Check sheet for the modelled part. Datum: model origin and axes. Units: mm. A direction names the side the tool comes from. Coordinates: 2 decimals unless noted, no trailing zeros. Loops run counter-clockwise (first coordinate to the right, second up) from the corner with the lowest first, then second, coordinate; pieces in that order, holes last. Notation, with made-up numbers: (-1, 32.25) - (8, 32.25) arc R29 cw to (8, 66.25) - close; hole circle Ø5 at (15, 75). An arc over 180 degrees is marked (long way). Write each question's results on one line, items separated by ' | '. Start each with the question number.
1. Gauge pin test, flat ends, axial feed: P1, Ø6, axis at x = 4.5, z = 14.5, coming from the +Y side; P2, Ø8, axis at x = 7.5, y = -7, coming from the +Z side; P3, Ø12, axis at x = 5, y = -9.5, coming from the -Z side. Record the tip position at first contact, or that the pin passes through.
2. Tool access check on faces 1 (the face through (11, 18, 40)), 2 (the face through (7.385, 0.751, -3.698)). Record the directions out of +Z, -Z, +X, -X, +Y, -Y that give a thin tool (end or side, any length) a straight path to the whole face; none if there is none.
3. Thickness scan on line 1 (Z direction, x = -13, y = 6.5); line 2 (Z direction, x = 7, y = 9); line 3 (X direction, y = 0.5, z = 20). Record the ranges inside material, lowest first. Write a range as [from, to].
4. Cross-section at B-B (z = 19). Record the cut outline in (x, y), and give its area (3 significant figures).
5. Cross-section at A-A (z = -3). Record the cut outline in (x, y), and give its area (3 significant figures).
```python
from build123d import *


with BuildPart() as f1:
    # F0 (on Front) → F1 (revolve)
    with BuildSketch(Plane.XZ):
        Polygon((10, 35), (5, 35), (5, -7.5), (7.5, -7.5), (7.5, 0), (10, 0), align=None)
        with BuildLine():
            Line((5, 37), (5, 35))
            Line((5, 35), (10, 35))
            Line((10, 35), (25, 35))
            Line((25, 35), (25, 40))
            Line((25, 40), (23.734994, 40))
            ThreePointArc((23.734994, 40), (14.486833, 37.754747), (5, 37))
        make_face()
    revolve(axis=Axis((5, 0, 14.75), (0, 0, 1)))


solid = f1.part
```
Established:
1) P1: y = 5 | P2: z = 38.1 | P3: z = 0
2) face 1: +Z, +X, -X, +Y, -Y | face 2: -Z
3) line 1: [35, 40] | line 2: [35, 37.71] | line 3: [0.03, 9.97]
4) outline: circle Ø10 at (5, 0) | area: 78.5 mm^2
5) outline: circle Ø5 at (5, 0) | area: 19.6 mm^2
